CAD build for the part. Positions are in the model's coordinates, mm. Coordinates: 2 decimals unless noted, no trailing zeros. Loops run counter-clockwise (first coordinate to the right, second up) from the corner with the lowest first, then second, coordinate; pieces in that order, holes last. Notation, with made-up numbers: M -16,32.5 L 2,32.5 A29 ccw 2,53.5 Z; hole C 9.5,46 d10. An arc over 180 degrees is marked long. Answer as a JSON object with one key per item and string values. Group by question number.
```python
from build123d import *

# Parameters (mm, degrees)
F0_W          = 66.5
F0_H          = 16.5
F1_DEPTH      = 0.8
F2_R          = 0.5
F3_DEPTH      = 17.7
F3_DEPTH_BACK = 33.25


with BuildPart() as f1:
    # F0 (on Top) → F1 (new body)
    with BuildSketch(Plane.XY):
        with Locations((33.25, 8.25)):
            Rectangle(F0_W, F0_H)
    extrude(amount=F1_DEPTH)

    # F2 (on face) → F3 (join, two sides)
    with BuildSketch(Plane.YZ.offset(66.5)) as f3_sk:
        with Locations((8.25, 1.2)):
            Circle(F2_R)
    extrude(amount=F3_DEPTH)
    extrude(f3_sk.sketch, amount=-F3_DEPTH_BACK)


solid = f1.part
```
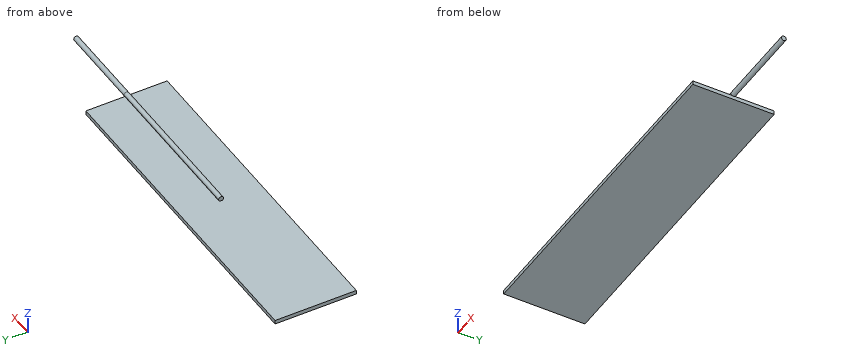
Item 1: Slice it at D-D, the plane x = 68. Write the cut outline in (y, z).
Item 2: Slice it at C-C, the plane x = 8.5. Write the cut outline in (y, z).
Item 3: Drill centre lines: L1, parallel to X at y = 5, z = 0.65; L2, parallel to Z at x = 54, y = 2.5; L3, parallel to Y at x = 69.5, z = 1.2. Where is each one in solid material? Low to high. Write a range as from..to.
Item 4: Pin check, flat tips, straight feed: pin 1 (5 mm diameter, centred on x = 14, y = 7, fed in from +Z); pin 2 (0.6 mm diameter, centred on y = 11.5, z = 0.5, fed in from +X). Stop position of each tip, or through.
Item 5: Slice it at B-B, the plane y = 4. Write the cut outline in (x, z).
Item 6: Slice it at A-A, the plane x = 50.5. Write the cut outline in (y, z), then the cut area to 3 significant figures.
Computed:
{
 "1": {"outline": "C 8.25,1.2 d1"},
 "2": {"outline": "M 0,0 L 16.5,0 L 16.5,0.8 L 0,0.8 Z"},
 "3": {"L1": "0..66.5", "L2": "0..0.8", "L3": "7.75..8.75"},
 "4": {"pin 1": "z = 0.8", "pin 2": "x = 66.5"},
 "5": {"outline": "M 0,0 L 66.5,0 L 66.5,0.8 L 0,0.8 Z"},
 "6": {"outline": "M 0,0 L 16.5,0 L 16.5,0.8 L 8.55,0.8 A0.5 ccw long 7.95,0.8 L 0,0.8 Z", "area": "13.9 mm2"}
}
